from build123d import *

# Parameters (mm, degrees)
BOSS_EXTRUDE1_DEPTH = 2
SKETCH2_R           = 3.2
CUT_EXTRUDE1_DEPTH  = 2
SKETCH5_R           = 2
CUT_EXTRUDE2_DEPTH  = 2
SKETCH10_R          = 2
CUT_EXTRUDE4_DEPTH  = 2


with BuildPart() as part:
    # Sketch1 → Boss-Extrude1 (new body)
    with BuildSketch(Plane.XY):
        with BuildLine():
            Line((0, 5), (330, 5))
            ThreePointArc((330, 5), (335, 0), (330, -5))
            Line((330, -5), (0, -5))
            ThreePointArc((0, -5), (-5, 0), (0, 5))
        make_face()
    extrude(amount=BOSS_EXTRUDE1_DEPTH)

    # Sketch2 → Cut-Extrude1 (cut)
    with BuildSketch(Plane.XY.offset(2)):
        with Locations((323, 0)):
            Circle(SKETCH2_R)
    extrude(amount=-CUT_EXTRUDE1_DEPTH, mode=Mode.SUBTRACT)

    # Sketch5 → Cut-Extrude2 (cut)
    with BuildSketch(Plane.XY.offset(2)):
        with Locations((190, 0)):
            Circle(SKETCH5_R)
        with Locations((170, 0)):
            Circle(SKETCH5_R)
        with Locations((150, 0)):
            Circle(SKETCH5_R)
        with Locations((130, 0)):
            Circle(SKETCH5_R)
    extrude(amount=-CUT_EXTRUDE2_DEPTH, mode=Mode.SUBTRACT)

    # Sketch10 → Cut-Extrude4 (cut)
    with BuildSketch(Plane.XY.offset(2)):
        Circle(SKETCH10_R)
    extrude(amount=-CUT_EXTRUDE4_DEPTH, mode=Mode.SUBTRACT)


solid = part.part
For this review, take the finished solid that the model builds, in its own axes (mm). Give positions to 0.01 mm unless a question says otherwise; leave off trailing zeros. Loops run counter-clockwise (first coordinate to the right, second up) from the corner with the lowest first, then second, coordinate; pieces in that order, holes last.
Item 1: Draft analysis for pull direction Y (two halves, no side actions). For faces 1 (the cylindrical face through (325.956, -1.226, 1.014)), 2 (the flat face through (167, 0, 2)), state which applies: +Y half, -Y half, draft (parallel to the pull), parting line (faces both ways), or undercut.
Item 2: Insertion check: pin 1 (1 mm diameter, centred on y = 1.5, z = 1.5, fed in from -X). The pin has a flat end and moves straight along its axis. Give the tip position at first contact, or say it passes through.
Item 3: Take a section at A-A, the plane x = 323. State the section outline as (y, z) points.
Item 4: For line 1 along Y through (x, z) = (0, 1.25); line 2 along Y through (x, z) = (323, 1.55); line 3 along X through (y, z) = (2.75, 1.6), list the stretches that pass through material, from the lowest coordinate up.
Item 5: Take a section at B-B, the plane z = 1.5. State the section outline as (x, y) points.
Calculated:
1. face 1: undercut
1. face 2: draft
2. pin 1: stops at x = -4.9
3. outline: (-5, 0) - (-3.2, 0) - (-3.2, 2) - (-5, 2) - close; (3.2, 0) - (5, 0) - (5, 2) - (3.2, 2) - close
4. line 1: y = -5 to -2, 2 to 5
4. line 2: y = -5 to -3.2, 3.2 to 5
4. line 3: x = -4.18 to 321.36, 324.64 to 334.18
5. outline: (0, -5) - (330, -5) arc R5 ccw to (330, 5) - (0, 5) arc R5 ccw to start; hole circle Ø4 at (0, 0); hole circle Ø4 at (130, 0); hole circle Ø4 at (150, 0); hole circle Ø4 at (170, 0); hole circle Ø4 at (190, 0); hole circle Ø6.4 at (323, 0)
